CAD build for the part. Positions are in the model's coordinates, mm. Face numbers are marked on the shaded views. A direction names the side the tool comes from. Give positions to 0.01 mm unless a question says otherwise; leave off trailing zeros. Order: outer loops, then holes, each group sorted by start corner. A loop starts at its lowest first (then second) coordinate and runs counter-clockwise, first axis right, second up.
Item 1: Wall check: L1, parallel to Z at x = -1.25, y = 2.25; L2, parallel to X at y = -1.75, z = -4.75; L3, parallel to X at y = 0.25, z = -17.25. Give the ranges that are in metal, low to high.
Item 2: Which spindle directions (+Z, -Z, +X, -X, +Y, -Y) get a long thin tool onto all of the face, cutting with end or side? Do the marked faces 1 and 2. Say none if no direction does.
Item 3: Band-saw the part on A-A on z = 0.5. Give the cut face in (x, y).
Item 4: Flat gauge pins, fed straight in: P1, Ø1.5, axis at y = -1.5, z = -4, coming from the -X side; P2, Ø1.5, axis at x = 0, z = -1.5, coming from the +Y side. Where does each tip first touch, or does it go through?
Item 5: Band-saw the part on B-B on z = -8.5. Give the cut face in (x, y).
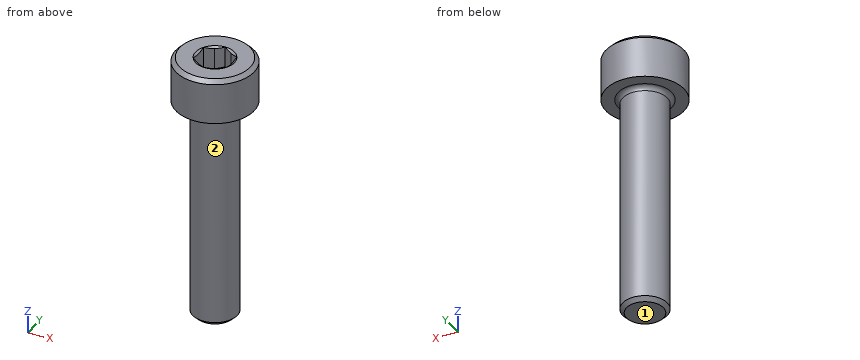
```python
from build123d import *

# Parameters (mm, degrees)
CHAMFER1_SIZE      = 0.35
CUT_EXTRUDE1_START = -2.000000153
CUT_EXTRUDE1_DEPTH = 3.000000153
FILLET2_R          = 0.4


with BuildPart() as part:
    # Sketch1 → Revolve1 (revolve)
    with BuildSketch(Plane(origin=(0, 0, 0), x_dir=(0, 0, -1), z_dir=(1, 0, 0)), mode=Mode.PRIVATE) as revolve1_sk:
        Polygon((0, 3.5), (-4, 3.5), (-4, 0), (20, 0), (20, 2), (0, 2), align=None)
    revolve(revolve1_sk.sketch.rotate(Axis((0, 0, 4), (0, 0, -1)), 180), axis=Axis((0, 0, 4), (0, 0, -1)))

    # Sketch7 → Cut-Revolve2 (revolve, cut)
    with BuildSketch(Plane(origin=(0, 0, 0), x_dir=(0, 0, -1), z_dir=(1, 0, 0)), mode=Mode.PRIVATE) as cut_revolve2_sk:
        Polygon((-4, 0), (-4, 1.5), (-2, 1.5), (-1.133974596, 0), align=None)
    revolve(cut_revolve2_sk.sketch.rotate(Axis((0, 0, 4), (0, 0, -1)), 90), axis=Axis((0, 0, 4), (0, 0, -1)), mode=Mode.SUBTRACT)

    # Chamfer1
    chamfer1_edges = [part.edges().sort_by_distance(p)[0] for p in [
        (0, 3.5, 4),
        (0, 2, -20),
    ]]
    chamfer(chamfer1_edges, length=CHAMFER1_SIZE)

    # Cut-Extrude1: read off the stored shape, not the designer's step
    # Cut-Extrude1 outline → Cut-Extrude1 (cut)
    with BuildSketch(Plane.XY.offset(4).offset(CUT_EXTRUDE1_START)):
        with BuildLine():
            Line((1.5, 0), (1.5, 0.866025404))
            Line((1.5, 0.866025404), (0.750000011, 1.299038099))
            ThreePointArc((0.750000011, 1.299038099), (1.299038109, 0.749999994), (1.5, 0))
        make_face()
        with BuildLine():
            ThreePointArc((-0.749999993, 1.29903811), (1e-08, 1.5), (0.750000011, 1.299038099))
            Line((0.750000011, 1.299038099), (0, 1.732050808))
            Line((0, 1.732050808), (-0.749999993, 1.29903811))
        make_face()
        with BuildLine():
            Line((1.5, -0.866025404), (1.5, 0))
            ThreePointArc((1.5, 0), (1.299038107, -0.749999997), (0.750000005, -1.299038103))
            Line((0.750000005, -1.299038103), (1.5, -0.866025404))
        make_face()
        with BuildLine():
            ThreePointArc((-1.5, 0), (-1.299038104, 0.750000003), (-0.749999993, 1.29903811))
            Line((-0.749999993, 1.29903811), (-1.5, 0.866025404))
            Line((-1.5, 0.866025404), (-1.5, 0))
        make_face()
        with BuildLine():
            Line((0, -1.732050808), (0.750000005, -1.299038103))
            ThreePointArc((0.750000005, -1.299038103), (3e-09, -1.5), (-0.75, -1.299038106))
            Line((-0.75, -1.299038106), (0, -1.732050808))
        make_face()
        with BuildLine():
            ThreePointArc((-0.75, -1.299038106), (-1.299038106, -0.75), (-1.5, 0))
            Line((-1.5, 0), (-1.5, -0.866025404))
            Line((-1.5, -0.866025404), (-0.75, -1.299038106))
        make_face()
    extrude(amount=CUT_EXTRUDE1_DEPTH, mode=Mode.SUBTRACT)

    # Cut-Extrude1 2 outline → Cut-Extrude1 2 (revolve)
    with BuildSketch(Plane.XZ):
        Polygon((1.732050916, 2.133974659), (1.499999934, 1.999999962), (1.732050808, 1.999999847), align=None)
    revolve(axis=Axis((0, 0, 0), (0, 0, 1)))

    # Sketch9 → Cut-Revolve3 (revolve, cut)
    with BuildSketch(Plane(origin=(0, 0, 0), x_dir=(0, 0, -1), z_dir=(1, 0, 0))):
        Polygon((-4.5, 2.598076211), (-4.5, 1.5), (-3.866025404, 1.5), align=None)
    revolve(axis=Axis((0, 0, 4), (0, 0, -1)), mode=Mode.SUBTRACT)

    # Fillet2
    fillet2_edges = [part.edges().sort_by_distance(p)[0] for p in [
        (0, 2, 0),
    ]]
    fillet(fillet2_edges, radius=FILLET2_R)


solid = part.part
```
The answers:
1. L1: z = 0 to 4
1. L2: x = -0.97 to 0.97
1. L3: x = -1.98 to 1.98
2. face 1: -Z, +X, -X, +Y, -Y
2. face 2: -Z
3. outline: circle Ø7 at (0, 0)
4. P1: stops at x = -1.85
4. P2: stops at y = 2
5. outline: circle Ø4 at (0, 0)
